Autodesk Inventor part; units mm, degrees
ref_plane "YZ Plane" through (0, 0, 0) normal (1, 0, 0) x (0, 1, 0)
ref_plane "XZ Plane" through (0, 0, 0) normal (0, 1, 0) x (-1, 0, 0)
ref_plane "XY Plane" through (0, 0, 0) normal (0, 0, 1) x (1, 0, 0)
sketch "Sketch1" plane through (0, 0, 0) normal (0, 1, 0) x (-1, 0, 0)
  line L0 (5.1091, 27.5) -> (-62.3909, 27.5)
  line L1 (-62.3909, 27.5) -> (-62.3909, -15)
  line L2 (-62.3909, -15) -> (5.1091, -15)
  line L3 (5.1091, -15) -> (5.1091, 27.5)
  line L4 (5.1091, 6.25) -> (-62.3909, 6.25)
  point P0 (0, 0)
  dimension "d0" = 42.5
  dimension "d1" = 67.5
extrude "Extrusion1" add sketch "Sketch1" along normal blind 5.31
sketch "Sketch2" plane through (0, 5.31, 0) normal (0, 1, 0) x (1, 0, 0)
  circle A0 centre (9.9709, -6.25) radius 0.75
  circle A1 centre (15.6009, -13.28) radius 0.75
  circle A2 centre (15.6009, 0.78) radius 0.75
  circle A3 centre (47.3109, -6.25) radius 0.75
  line L0 (-5.1091, -6.25) -> (62.3909, -6.25) construction
  line L1 (15.6009, 15.6122) -> (15.6009, -24.3614) construction
  line L2 (11.7209, -11.53) -> (45.5609, -11.53)
  line L3 (45.5609, -11.53) -> (45.5609, -0.97)
  line L4 (45.5609, -0.97) -> (11.7209, -0.97)
  line L5 (11.7209, -0.97) -> (11.7209, -11.53)
  circle A4 centre (-0.8591, 10.75) radius 1.75
  line L6 (62.3909, 15) -> (-5.1091, 15)
  circle A5 centre (-0.8591, -23.25) radius 1.75
  line L7 (-5.1091, -27.5) -> (62.3909, -27.5)
  circle A6 centre (58.1409, 10.75) radius 1.75
  circle A7 centre (58.1409, -23.25) radius 1.75
  line L8 (62.3909, -27.3764) -> (62.3909, 12.6236)
  line L9 (28.6409, -27.5) -> (28.6409, 15) construction
  line L10 (62.3909, -27.5) -> (62.3909, 15)
  line L11 (-5.1091, -27.5) -> (62.3909, -27.5)
  line L12 (-5.1091, 15) -> (-5.1091, -27.5)
  line L13 (62.3909, 15) -> (-5.1091, 15)
  point P0 (0, 0)
  dimension "d4" = 1.5
  dimension "d15" = 14.06
  dimension "d23" = 37.34
  dimension "d39" = 5.63
  dimension "d70" = 4.25
  dimension "d79" = 3.5
  dimension "d90" = 4.25
  dimension "d91" = 4.25
  dimension "d93" = 34
  dimension "d94" = 59
  dimension "d101" = 1
  dimension "d102" = 1
  dimension "d103" = 1
  dimension "d105" = 1
extrude "Extrusion2" cut sketch "Sketch2" against normal through all contours A0 | A1 | A2 | A3 | L5 L4 L3 L2 | A4 | A5 | A6 | A7
sketch "Sketch4" plane through (0, 5.31, 0) normal (0, 1, 0) x (1, 0, 0)
  circle A0 centre (-0.8591, 10.75) radius 3.75
  circle A1 centre (58.1409, -23.25) radius 3.75
  circle A2 centre (58.1409, 10.75) radius 3.75
  circle A3 centre (-0.8591, -23.25) radius 3.75
  circle A4 centre (-0.8591, -23.25) radius 1.75 construction
  circle A5 centre (58.1409, -23.25) radius 1.75 construction
  circle A6 centre (-0.8591, 10.75) radius 1.75 construction
  circle A7 centre (58.1409, 10.75) radius 1.75 construction
  circle A8 centre (58.1409, -23.25) radius 1.75
  circle A9 centre (-0.8591, -23.25) radius 1.75
  circle A10 centre (-0.8591, 10.75) radius 1.75
  circle A11 centre (58.1409, 10.75) radius 1.75
  circle A12 centre (47.5609, -13.53) radius 1
  circle A13 centre (9.7209, -13.53) radius 1
  circle A14 centre (47.5609, 1.03) radius 1
  circle A15 centre (9.7209, 1.03) radius 1
  line L0 (45.5609, -11.53) -> (11.7209, -11.53)
  line L1 (45.5609, -0.97) -> (45.5609, -11.53)
  line L2 (28.6409, -33.9575) -> (28.6409, 25.5773) construction
  line L3 (71.7292, -6.25) -> (-26.8251, -6.25) construction
  line L4 (47.5609, -13.53) -> (9.7209, -13.53) construction
  line L5 (47.5609, 1.03) -> (9.7209, 1.03) construction
  circle A16 centre (28.6409, 1.03) radius 1
  circle A17 centre (28.6409, -13.53) radius 1
  point P0 (0, 0)
  point P1 (56.8909, 12)
  point P2 (-2.1091, 12)
  dimension "d92" = 2
  dimension "d95" = 2
  dimension "d96" = 2
  dimension "d97" = 2
extrude "Extrusion4" add sketch "Sketch4" along normal blind 2
sketch "Sketch5" plane through (58.1409, 7.31, -10.75) normal (0, 1, 0) x (1, 0, 0)
  circle A0 centre (0, -34) radius 1.75
  circle A1 centre (0, -34) radius 1
  circle A2 centre (0, -34) radius 3.75
  circle A3 centre (-59, -34) radius 1.75
  circle A4 centre (-59, -34) radius 1.75
  circle A5 centre (-59, -34) radius 3.75
  circle A6 centre (-59, -34) radius 1.75
  circle A7 centre (-59, -34) radius 3.75
  circle A8 centre (0, -34) radius 3.75
  circle A9 centre (-59, 0) radius 1.75
  circle A10 centre (0, 0) radius 1.75
  circle A11 centre (-59, 0) radius 3.75
  circle A12 centre (0, 0) radius 3.75
  circle A13 centre (0, 0) radius 3.75
  circle A14 centre (0, 0) radius 1.75
  circle A15 centre (-59, 0) radius 1.75
  circle A16 centre (-59, 0) radius 3.75
  point P0 (-58.1409, -10.75)
extrude "Extrusion5" add sketch "Sketch5" along normal blind 2.3 contours A2 | A5 | A11 | A12
equation "\"d31\" = d69"
properties part number "490HV_MicrofluidicClamp"
The listing builds one solid part. Answer for the finished solid, in the listing's coordinates (mm). A direction names the side the tool comes from. Give positions to 0.01 mm unless a question says otherwise; leave off trailing zeros. Write each loop counter-clockwise with the first axis right and the second up, starting at its lowest first coordinate (ties: lowest second). Pieces come first, ordered by that corner, then holes. Notation, with made-up numbers: (55.25, -28.5) - (103.25, -28.5) arc R25 ccw to (103.25, -14.5) - close; hole circle Ø3 at (73.5, 47.25). An arc over 180 degrees is marked (long way). Use one line per item in the form item = value. Start each with the question number.
1) Flat-ended cylindrical pins translate along their axes: pin 1 Ø10 at (x, z) = (29, -8) entering from +Y; pin 2 Ø1.2 at (x, z) = (15.6, -0.78) entering from -Y; pin 3 Ø1 at (x, z) = (48, -0.5) entering from +Y; pin 4 Ø2 at (x, y) = (3.5, 6.5) entering from -Z. Find the tip coordinate at first contact, or state that the pin passes through.
2) Find section B-B on x = 21.5. Determine the outline of the cut face in (y, z), plus the area to 3 significant figures.
3) Find section C-C on z = 6.25. Determine the outline of the cut face in (x, y).
4) The mould has two halves that part along X. Classify faces 1 (the face through (11.721, 3, 6)), 2 (the face through (10, 7.31, 14)), 3 (the face through (62.391, 3, 7)): pulls with the +X half, pulls with the -X half, needs draft (parallel to the pull), parting line crosses it, or undercut.
5) A tool of negligible diameter and unlimited length cuts with its end or side. For faces 4 (the face through (29.18, 6.3, 14.37)), 5 (the face through (29, 7.31, -1)), from which of +Z, -Z, +X, -X, +Y, -Y can it reach the whole face along a straight path? Write none if from no direction.
6) Consider line 1 along X through (y, z) = (5.5, 23.25); line 2 along X through (y, z) = (2.2, 6.25); line 3 along Z through (x, y) = (58, 9). Determine where each line is inside the solid, lowest interval first. Write a range as from..to.
7) Find section A-A on z = 23.25. Determine the outline of the cut face in (x, y), plus the area to 3 significant figures.
8) Find section D-D on y = 2.5. Count the separate pieces of the cut face and the enclosed holes in it, plus the area to 3 significant figures.
Geometry results:
q1.pin_1 = 5.31
q1.pin_2 = through
q1.pin_3 = 7.31
q1.pin_4 = -12.42
q2.outline = (0, -15) - (5.31, -15) - (5.31, 0.97) - (0, 0.97) - close; (0, 11.53) - (5.31, 11.53) - (5.31, 27.5) - (0, 27.5) - close
q2.area = 170 mm2
q3.outline = (-5.11, 0) - (9.22, 0) - (9.22, 5.31) - (-5.11, 5.31) - close; (10.72, 0) - (11.72, 0) - (11.72, 5.31) - (10.72, 5.31) - close; (45.56, 0) - (46.56, 0) - (46.56, 5.31) - (45.56, 5.31) - close; (48.06, 0) - (62.39, 0) - (62.39, 5.31) - (48.06, 5.31) - close
q4.face_1 = undercut
q4.face_2 = needs draft
q4.face_3 = pulls with the +X half
q5.face_4 = +Y
q5.face_5 = +Z, -Z, +X, -X, +Y
q6.line_1 = -4.61..-2.61, 0.89..2.89, 54.39..56.39, 59.89..61.89
q6.line_2 = -5.11..9.22, 10.72..11.72, 45.56..46.56, 48.06..62.39
q6.line_3 = -14.5..-12.49, -9.01..-7, 19.5..21.51, 24.99..27
q7.outline = (-5.11, 0) - (-2.61, 0) - (-2.61, 9.61) - (-4.61, 9.61) - (-4.61, 5.31) - (-5.11, 5.31) - close; (0.89, 0) - (56.39, 0) - (56.39, 9.61) - (54.39, 9.61) - (54.39, 5.31) - (2.89, 5.31) - (2.89, 9.61) - (0.89, 9.61) - close; (59.89, 0) - (62.39, 0) - (62.39, 5.31) - (61.89, 5.31) - (61.89, 9.61) - (59.89, 9.61) - close
q7.area = 356 mm2
q8.separate_pieces = 1
q8.enclosed_holes = 9
q8.area = 2,470 mm2
